Autodesk Inventor part; units mm, degrees
ref_plane "YZ Plane" through (0, 0, 0) normal (1, 0, 0) x (0, 1, 0)
ref_plane "XZ Plane" through (0, 0, 0) normal (0, 1, 0) x (-1, 0, 0)
ref_plane "XY Plane" through (0, 0, 0) normal (0, 0, 1) x (1, 0, 0)
sketch "Sketch1" plane through (0, 0, 0) normal (0, 0, 1) x (1, 0, 0)
  circle A0 centre (0, 0) radius 45
  circle A1 centre (0, 0) radius 30
  circle A2 centre (0, 37.5) radius 4
  circle A3 centre (-37.5, 0) radius 4
  circle A4 centre (0, -37.5) radius 4
  circle A5 centre (37.5, 0) radius 4
  dimension "d0" = 90
  dimension "d1" = 60
  dimension "d2" = 8
  dimension "d3" = 37.5
  dimension "d6" = 360
  dimension "d8" = 75
  dimension "d9" = 37.5
  dimension "d10" = 37.5
  dimension "d11" = 75
extrude "Extrusion1" add sketch "Sketch1" along normal mid plane 1
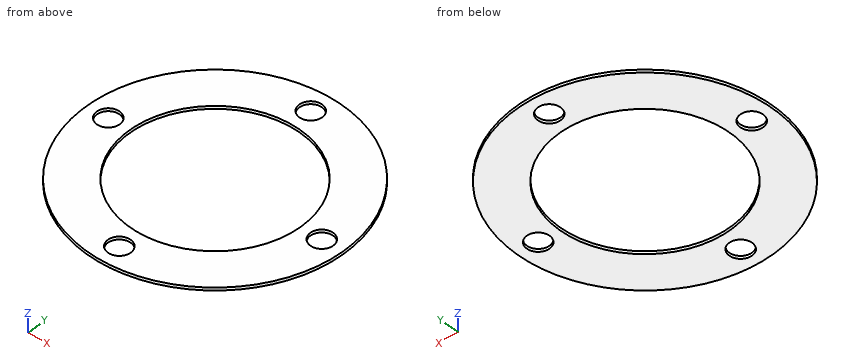
Work out the finished part from the listing and answer in its coordinate system (mm). Give positions to 0.01 mm unless a question says otherwise; leave off trailing zeros. Order: outer loops, then holes, each group sorted by start corner. A loop starts at its lowest first (then second) coordinate and runs counter-clockwise, first axis right, second up. Notation, with made-up numbers: M 9.5,61 L 22.5,61 A26 ccw 22.5,80 Z; hole C 80,55 d2. An arc over 180 degrees is marked long. Return JSON: item names as keys, results as strings.
Q1. Find section B-B, the plane y = -39.5. Write down the section's boundary in (x, z), and give its area (3 significant figures).
Answer below:
{"outline": "M -21.56,-0.5 L -3.46,-0.5 L -3.46,0.5 L -21.56,0.5 Z; M 3.46,-0.5 L 21.56,-0.5 L 21.56,0.5 L 3.46,0.5 Z", "area": "36.2 mm^2"}
Q2. Find section D-D, the plane x = -15. Write down the section's boundary in (y, z), and give its area (3 significant figures).
Answer below:
{"outline": "M -42.43,-0.5 L -25.98,-0.5 L -25.98,0.5 L -42.43,0.5 Z; M 25.98,-0.5 L 42.43,-0.5 L 42.43,0.5 L 25.98,0.5 Z", "area": "32.9 mm^2"}
Q3. Find section C-C, the plane z = 0. Write down the section's boundary in (x, y).
Answer below:
{"outline": "C 0,0 d90; hole C -37.5,0 d8; hole C 0,0 d60; hole C 0,-37.5 d8; hole C 0,37.5 d8; hole C 37.5,0 d8"}
Q4. Find section A-A, the plane x = 0. Write down the section's boundary in (y, z).
Answer below:
{"outline": "M -45,-0.5 L -41.5,-0.5 L -41.5,0.5 L -45,0.5 Z; M -33.5,-0.5 L -30,-0.5 L -30,0.5 L -33.5,0.5 Z; M 30,-0.5 L 33.5,-0.5 L 33.5,0.5 L 30,0.5 Z; M 41.5,-0.5 L 45,-0.5 L 45,0.5 L 41.5,0.5 Z"}
Q5. Find the intervals of material crossed by line 1 along Y through (x, z) = (0, 0.1); line 2 along Y through (x, z) = (-2, 0.25); line 3 along Y through (x, z) = (-15, -0.35), in increasing order. Write a range as [from, to].
Answer below:
{"line 1": "y = [-45, -41.5], [-33.5, -30], [30, 33.5], [41.5, 45]", "line 2": "y = [-44.96, -40.96], [-34.04, -29.93], [29.93, 34.04], [40.96, 44.96]", "line 3": "y = [-42.43, -25.98], [25.98, 42.43]"}
